Design review of the part built by this model. Coordinates are the model's own, in mm. A direction names the side the tool comes from. Coordinates: 2 decimals unless noted, no trailing zeros. Loops run counter-clockwise (first coordinate to the right, second up) from the corner with the lowest first, then second, coordinate; pieces in that order, holes last. Notation, with made-up numbers: (3.25, 8) -> (24.25, 8) arc R17 ccw to (24.25, 31) -> close; hole circle Ø11 at (6, 39). An arc over 180 degrees is marked (long way). Use a Markdown table: item, result. Add a question column.
Q1. Take a section at C-C on y = 28. Write out the cut boundary in (x, z), plus the area to 3 significant figures.
Q2. Take a section at B-B on z = -8. Write out the cut boundary in (x, y).
Q3. Draft analysis for pull direction Y (two halves, no side actions). For faces 1 (the face through (0, 20, -4)), 2 (the face through (-1.782, 17.727, -8.358)), 3 (the face through (0, 0, -7)), state which applies: pulls with the +Y half, pulls with the -Y half, needs draft (parallel to the pull), parting line crosses it, or undercut.
Q4. For faces 4 (the face through (-0.314, 4.93, -12.916)), 5 (the face through (-0.314, 25.07, -2.084)), 6 (the face through (-4.142, 17.788, -7.23)), 7 (the face through (4.5, 15, -8)), list the 3-axis set-ups (+Z, -Z, +X, -X, +Y, -Y) from which the entire face can be reached by the end or side of a thin tool; tool diameter is ignored.
Q5. For probe 1 along Z at (x, y) = (0, 25); probe 2 along Y at (x, z) = (3.2, -6.75); probe 3 along Y at (x, z) = (-2, -9), list the stretches that pass through material, from the lowest coordinate up.
Q6. Clearance check with flat-ended pins moving along their axes: pin 1 Ø1.7 at (x, z) = (0, -11.5) entering from +Y; pin 2 Ø1 at (y, z) = (6.5, -12) entering from +X; pin 3 Ø1 at (x, z) = (1, -5) entering from -Y. State where each tip first meets the part, or that it passes through.
Q7. Take a section at D-D on x = 3.25. Write out the cut boundary in (y, z).
Q8. Take a section at A-A on x = 0. Write out the cut boundary in (y, z), plus the area to 3 significant figures.
Autodesk Inventor part; units mm, degrees
ref_plane "YZ Plane" through (0, 0, 0) normal (1, 0, 0) x (0, 1, 0)
ref_plane "XZ Plane" through (0, 0, 0) normal (0, 1, 0) x (-1, 0, 0)
ref_plane "XY Plane" through (0, 0, 0) normal (0, 0, 1) x (1, 0, 0)
sketch "Sketch2" plane through (0, 0, 0) normal (0, 1, 0) x (-1, 0, 0)
  line L0 (-4.5, -10) -> (-4.5, -5)
  line L1 (4.5, -10) -> (4.5, -5)
  arc A0 (4.5, -5) -> (-4.5, -5) centre (0, -5) ccw
  arc A1 (-4.5, -10) -> (4.5, -10) centre (0, -10) ccw
  point P0 (0, 0)
  point P1 (0.9888, -13.1808)
  dimension "d75" = 5
  dimension "d76" = 5
extrude "Extrusion1" add sketch "Sketch2" along normal blind 30
sketch "Sketch14" plane through (-4.5, 0, -10) normal (-1, 0, 0) x (0, 0, 1)
  line L0 (-4.5, 0) -> (-4.5, 30)
  line L1 (-4.5, 0) -> (-4.5, 15)
  line L2 (-4.5, 15) -> (2, 15)
  circle A0 centre (2, 15) radius 2.75
  point P0 (10, 0)
  point P1 (-11.5, 30)
  dimension "d80" = 15
  dimension "d81" = 6.5
  dimension "d82" = 5.5
extrude "Extrusion13" cut sketch "Sketch14" against normal blind 5 and the other way blind 5
sketch "Sketch18" plane through (0, 30, 0) normal (0, 1, 0) x (1, 0, 0)
  arc A0 (4.5, 10) -> (-4.5, 10) centre (0, 10) ccw
  line L0 (0, 14.5) -> (0, 11.5)
  circle A1 centre (0, 11.5) radius 1.45
  arc A2 (-4.5, 5) -> (4.5, 5) centre (0, 5) ccw
  line L1 (0, 0.5) -> (0, 3.5)
  circle A3 centre (0, 3.5) radius 1.45
  point P0 (0, 0)
  dimension "d103" = 3
  dimension "d104" = 2.9
  dimension "d105" = 3
  dimension "d106" = 2.9
extrude "Extrusion17" cut sketch "Sketch18" against normal blind 10
sketch "Sketch19" plane through (0, 0, 0) normal (0, -1, 0) x (1, 0, 0)
  line L0 (4.5, -10) -> (4.5, -5)
  arc A0 (4.5, -5) -> (-4.5, -5) centre (0, -5) ccw
  line L1 (-4.5, -5) -> (-4.5, -10)
  arc A1 (-4.5, -10) -> (4.5, -10) centre (0, -10) ccw
  circle A2 centre (0, -11.5) radius 1.45
  circle A3 centre (0, -3.5) radius 1.45
extrude "Extrusion18" cut sketch "Sketch19" against normal blind 10 contours A2 | A3
sketch "Sketch20" plane through (0.5, 15, -8) normal (-1, 0, 0) x (0, 0, 1)
  circle A0 centre (0, 0) radius 2.75
  line L0 (0, 0) -> (-1.25, 0)
  line L1 (0, 0) -> (1.25, 0) construction
  line L2 (0, 0) -> (1.25, 0)
  line L3 (0, 0) -> (1.25, 0) construction
  circle A1 centre (-1.25, 0) radius 0.8
  circle A2 centre (1.25, 0) radius 0.8
  point P0 (8, -15)
  dimension "d115" = 1.25
  dimension "d116" = 180
  dimension "d117" = 1.25
  dimension "d118" = 0
  dimension "d119" = 1.6
  dimension "d120" = 1.6
extrude "Extrusion19" cut sketch "Sketch20" against normal through all contours A1 | A2
chamfer "Chamfer5" distance 0.5 angle 45 3 edges at (-4.5, 12.4444, -6.9845) (-4.5, 17.5556, -6.9845) (-4.4371, 15.0001, -10.75)
properties part number "Front mount" material "ABS Plastic"
Answer list:
| question | item | result |
|---|---|---|
| 1 | outline | (-4.5, -10) arc R4.5 ccw to (4.5, -10) -> (4.5, -5) arc R4.5 ccw to (-4.5, -5) -> close; hole circle Ø2.9 at (0, -11.5); hole circle Ø2.9 at (0, -3.5) |
| 1 | area | 95.4 mm² |
| 2 | outline | (-4.5, 0) -> (4.5, 0) -> (4.5, 30) -> (-4.5, 30) -> (-4.5, 18.25) -> (-4, 17.75) -> (0.5, 17.75) -> (0.5, 12.25) -> (-4, 12.25) -> (-4.5, 11.75) -> close |
| 3 | face 1 | pulls with the +Y half |
| 3 | face 2 | undercut |
| 3 | face 3 | pulls with the -Y half |
| 4 | face 4 | -Y |
| 4 | face 5 | +Y |
| 4 | face 6 | -X |
| 4 | face 7 | +Z, -Z, +X, +Y, -Y |
| 5 | probe 1 | -14.5 to -12.95, -10.05 to -4.95, -2.05 to -0.5 |
| 5 | probe 2 | 0 to 14.2, 15.8 to 30 |
| 5 | probe 3 | 0 to 12.44, 17.56 to 30 |
| 6 | pin 1 | y = 20 |
| 6 | pin 2 | x = 4.24 |
| 6 | pin 3 | y = 0 |
| 7 | outline | (0, -13.11) -> (30, -13.11) -> (30, -1.89) -> (0, -1.89) -> close; hole circle Ø1.6 at (15, -9.25); hole circle Ø1.6 at (15, -6.75) |
| 8 | outline | (0, -14.5) -> (30, -14.5) -> (30, -12.95) -> (20, -12.95) -> (20, -10.05) -> (30, -10.05) -> (30, -4.95) -> (20, -4.95) -> (20, -2.05) -> (30, -2.05) -> (30, -0.5) -> (0, -0.5) -> (0, -2.05) -> (10, -2.05) -> (10, -4.95) -> (0, -4.95) -> (0, -10.05) -> (10, -10.05) -> (10, -12.95) -> (0, -12.95) -> close; hole circle Ø5.5 at (15, -8) |
| 8 | area | 280 mm² |
